Study the drawing (mm; zero at the part's minimum x, y, z) and answer. A direction names the side the tool comes from. Round coordinates to 2 decimals unless told otherwise and drop trailing zeros. Write each loop counter-clockwise with the first axis right and the second up, starting at its lowest first coordinate (ties: lowest second). Pieces come first, ordered by that corner, then holes.
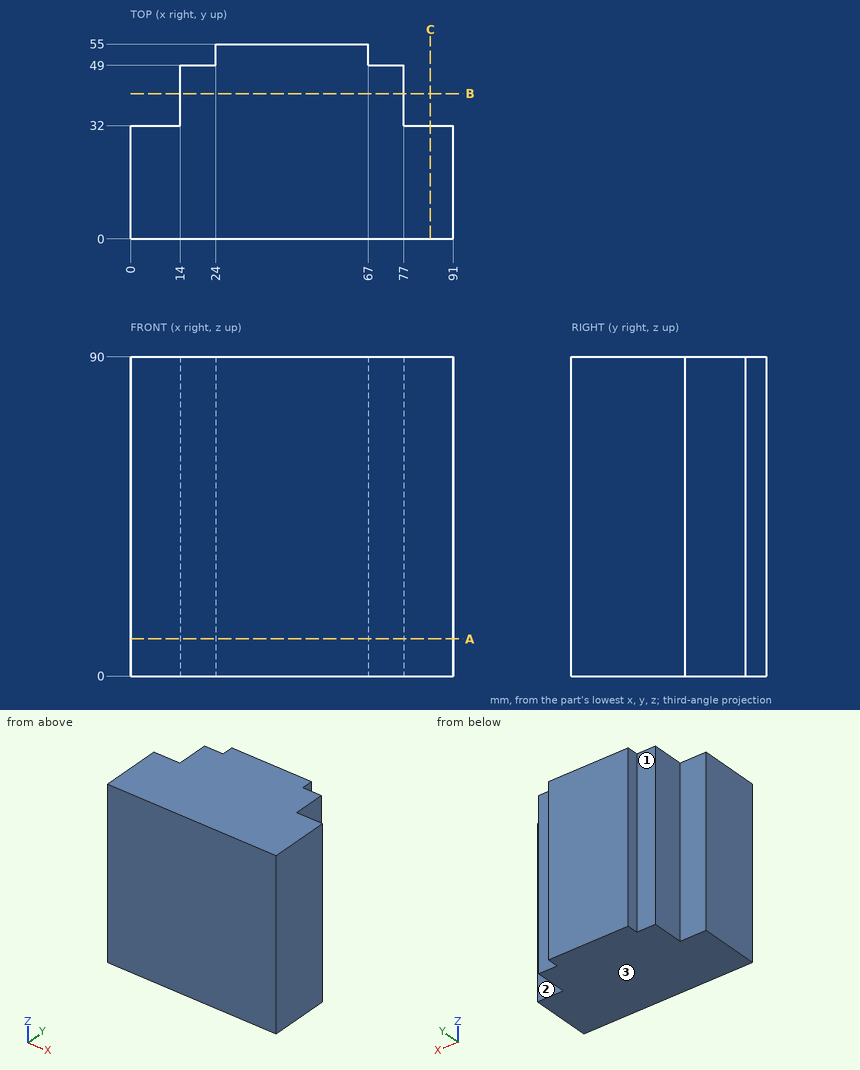
1. Straight lines are drawn through the part: line 1 along Y through (x, z) = (69, 24); line 2 along Y through (x, z) = (86, 48); line 3 along X through (y, z) = (37, 12). For each, find the intervals that lie inside material, in ascending order.
Geometry says:
line 1: y = 0 to 49
line 2: y = 0 to 32
line 3: x = 14 to 77
2. Section C-C on x = 84.5 is taken. Determine the outline of the cut face in (y, z), plus the area to 3 significant figures.
Geometry says:
outline: (0, 0) - (32, 0) - (32, 90) - (0, 90) - close
area: 2,880 mm2
3. Given pin 1 (6 mm diameter, centred on x = 42, z = 63, fed in from -Y); pin 2 (5 mm diameter, centred on y = 52.5, z = 42, fed in from -X); pin 3 (8.5 mm diameter, centred on y = 44, z = 56, fed in from -X); pin 4 (18.5 mm diameter, centred on y = 42.5, z = 46, fed in from +X), each flat-ended and moving along its own axis, determine where each tip first touches the part or whether it passes through.
Geometry says:
pin 1: stops at y = 0
pin 2: stops at x = 24
pin 3: stops at x = 14
pin 4: stops at x = 77
4. Section B-B on y = 41 is taken. Determine the outline of the cut face in (x, z), plus the area to 3 significant figures.
Geometry says:
outline: (14, 0) - (77, 0) - (77, 90) - (14, 90) - close
area: 5,670 mm2
5. Section A-A on z = 10.5 is taken. Determine the outline of the cut face in (x, y), plus the area to 3 significant figures.
Geometry says:
outline: (0, 0) - (91, 0) - (91, 32) - (77, 32) - (77, 49) - (67, 49) - (67, 55) - (24, 55) - (24, 49) - (14, 49) - (14, 32) - (0, 32) - close
area: 4,240 mm2
6. A tool of negligible diameter and unlimited length cuts with its end or side. For the marked faces 1, 2 and 3, from which of +Z, -Z, +X, -X, +Y, -Y can it reach the whole face along a straight path? Write none if from no direction.
Geometry says:
face 1: +Z, -Z, -X, +Y
face 2: +Z, -Z, +X, +Y
face 3: -Z, +X, -X, +Y, -Y
